```python
from build123d import *

# Parameters (mm, degrees)
F2_SIZE2       = 1.58749
F2_SIZE        = 6.34999
F3_SIZE2       = 1.58749
F3_SIZE        = 6.34999
F5_D           = 5.159375
F5_CSINK_D     = 11.1125
F5_CSINK_ANGLE = 90


# Not quite as in the source:
# - a fillet or chamfer is up to 0.001 mm smaller than in the source, because OpenCascade refuses the exact size


with BuildPart() as f1:
    # F0 (on Right) → F1 (revolve)
    with BuildSketch(Plane.YZ):
        Polygon((-15.875, 13.49375), (0, 13.49375), (0, 41.9197008275), (-3.175, 41.9197008275), (-3.175, 35.5697008275), (-12.7, 35.5697008275), (-12.7, 41.9197008275), (-15.875, 41.9197008275), align=None)
    revolve(axis=Axis((0, -7.9375, 0), (0, 1, 0)))

    # F2 (size 6.35 and 1.5875 in the source; OpenCascade refuses exactly that, so slightly less here)
    f2_edges = [f1.edges().sort_by_distance(p)[0] for p in [
        (0, -12.7, -41.919701),
    ]]
    f2_side = f1.faces().sort_by_distance((0, -12.7, -36.755369))[0]
    chamfer(f2_edges, length=F2_SIZE, length2=F2_SIZE2, reference=f2_side)

    # F3 (size 6.35 and 1.5875 in the source; OpenCascade refuses exactly that, so slightly less here)
    f3_edges = [f1.edges().sort_by_distance(p)[0] for p in [
        (0, -3.175, -41.919701),
    ]]
    chamfer(f3_edges, length=F3_SIZE, length2=F3_SIZE2)

    # F5 (through all)
    with Locations(Plane(origin=(0, 0, 0), x_dir=(-1, 0, 0), z_dir=(0, 1, 0))):
        with Locations((0, 22.606), (0, -22.606)):
            CounterSinkHole(F5_D / 2, F5_CSINK_D / 2, counter_sink_angle=F5_CSINK_ANGLE)


solid = f1.part
```
Read the model definition and answer for the solid it produces. Units are mm, in the model's axes. A direction names the side the tool comes from. Give positions to 0.01 mm unless a question says otherwise; leave off trailing zeros. Order: outer loops, then holes, each group sorted by start corner. A loop starts at its lowest first (then second) coordinate and runs counter-clockwise, first axis right, second up. Notation, with made-up numbers: (1.5, -14.75) -> (45.5, -14.75) arc R26 cw to (45.5, 22.25) -> close; hole circle Ø6 at (-33, 24). An arc over 180 degrees is marked (long way). Write item = value, one per line.
1. The mould has two halves that part along Y. Classify faces 1 (the face through (1.58, -12.8, -35.93)), 2 (the face through (-40.923, -15.092, -9.087)), 3 (the face through (2.6, -2.83, -21.79)): +Y half, -Y half, draft (parallel to the pull), parting line (faces both ways), or undercut.
Numbers:
face_1 = undercut
face_2 = draft
face_3 = +Y half
2. For faces 4 (the face through (29.993, -8.004, 19.122)), 5 (the face through (10, -15.875, -10)), determine the directions among +Z, -Z, +X, -X, +Y, -Y from which every point of the face is accessible in a straight line to the end or side of a thin tool.
Numbers:
face_4 = none
face_5 = +Z, -Z, +X, -X, -Y
3. Straight lines are drawn through the part: line 1 along Z through (x, y) = (2, -9.25); line 2 along Y through (x, z) = (25.5, 25) (3 decimals); line 3 along X through (y, z) = (-4.5, -7). For each, find the intervals that lie inside material, in ascending order.
Numbers:
line_1 = -35.51 to -24.24, -20.98 to -13.34, 13.34 to 20.98, 24.24 to 35.51
line_2 = -15.875 to -12.735, -3.14 to 0
line_3 = -34.87 to -11.54, 11.54 to 34.87
4. A cutting plane is placed at A-A, the plane x = 0. Count the separate pieces of the cut face and the enclosed holes in it, and give its area (3 significant figures).
Numbers:
separate_pieces = 4
enclosed_holes = 0
area = 580 mm²
5. Given pin 1 (8 mm diameter, centred on x = 22, y = -7, fed in from -Z); pin 2 (1 mm diameter, centred on x = -6.5, y = -10, fed in from -Z); pin 3 (1 mm diameter, centred on x = -8.5, y = -11, fed in from +Z); pin 4 (4 mm diameter, centred on x = 0, z = -22.606, fed in from +Y), each flat-ended and moving along its own axis, determine where each tip first touches the part or whether it passes through.
Numbers:
pin_1 = -30.68
pin_2 = -35.06
pin_3 = 34.66
pin_4 = through
6. A cutting plane is placed at C-C, the plane y = -11. Write down the section's boundary in (x, z).
Numbers:
outline = circle Ø71.14 at (0, 0); hole circle Ø26.99 at (0, 0); hole circle Ø5.16 at (0, -22.61); hole circle Ø5.16 at (0, 22.61)
